Check sheet for the drawn part. Datum: minimum x, y, z corner. Units: mm. Give positions to 0.01 mm unless a question says otherwise; leave off trailing zeros. Write each loop counter-clockwise with the first axis right and the second up, starting at its lowest first coordinate (ties: lowest second). Pieces come first, ordered by that corner, then holes. Notation, with made-up numbers: (45, 1) -> (49, 1) arc R14 cw to (49, 23) -> close; hole circle Ø6 at (56, 55.25). An arc over 180 degrees is marked (long way). Write item = value, one per line. Start each with the question number.
1. Depth check by flat-ended pin: P1, Ø2.5, axis at x = 7, y = 86.5, coming from the -Z side. Enter the tip coordinate at first touch or a pass-through.
2. Cross-section at A-A, the plane x = 7. Record the cut outline in (y, z), plus the area to 3 significant figures.
3. Thickness scan on line 1 along Y through (x, z) = (62.5, 2.75); line 2 along Y through (x, z) = (7, 1); line 3 along X through (y, z) = (86.5, 2.45). Record the ranges inside material, lowest first.
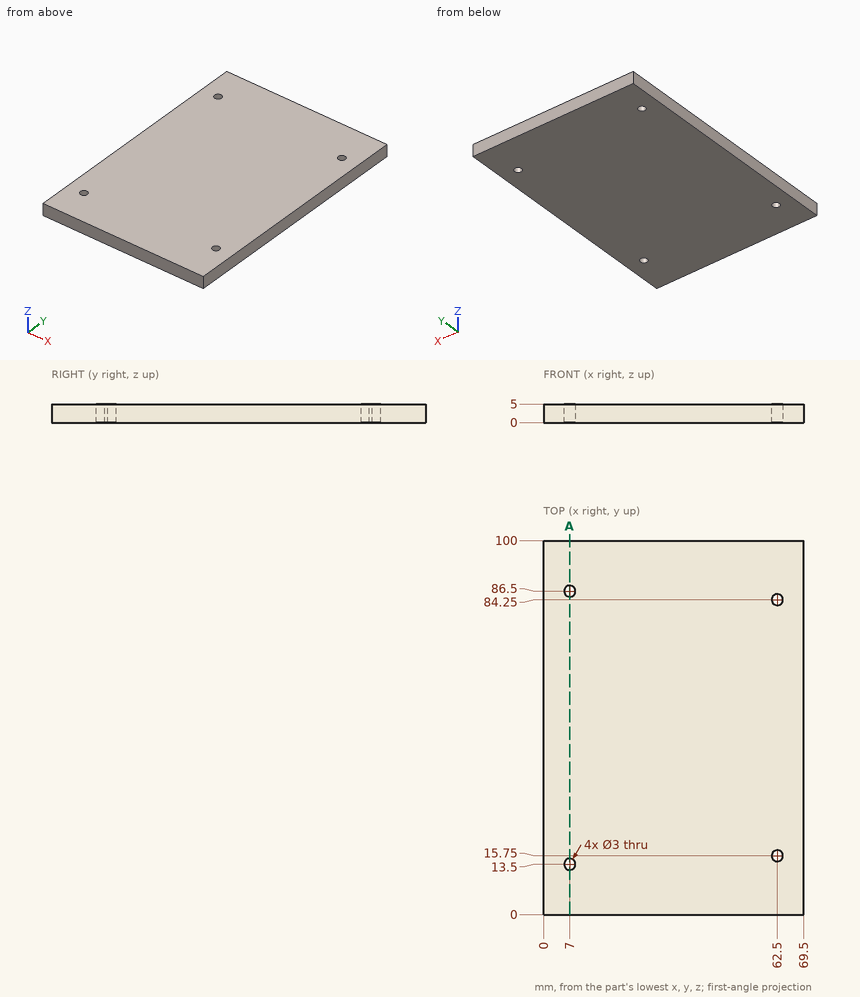
Answers:
q1.P1 = through
q2.outline = (0, 0) -> (12, 0) -> (12, 5) -> (0, 5) -> close; (15, 0) -> (85, 0) -> (85, 5) -> (15, 5) -> close; (88, 0) -> (100, 0) -> (100, 5) -> (88, 5) -> close
q2.area = 470 mm^2
q3.line_1 = 0 to 14.25, 17.25 to 82.75, 85.75 to 100
q3.line_2 = 0 to 12, 15 to 85, 88 to 100
q3.line_3 = 0 to 5.5, 8.5 to 69.5
